```python
from build123d import *

# Parameters (mm, degrees)
SKETCH_1_W                = 35
SKETCH_1_H                = 10
EXTRUDE_1_DEPTH           = 30
SKETCH_2_R                = 1.65
CUT_EXTRUDE_1_DEPTH       = 47.368092477
SKETCH_3_W                = 35
SKETCH_3_H                = 10
FILLET_1_R                = 5
SKETCH_6_W                = 70
SKETCH_6_H                = 60
EXTRUDE_2_DEPTH           = 10
CHAMFER_1_SIZE            = 10
CUT_EXTRUDE_3_DEPTH       = 15
SKETCH_8_R                = 15
CUT_EXTRUDE_4_DEPTH       = 15
SKETCH_10_R               = 2.1
CUT_EXTRUDE_6_DEPTH       = 156.505811286
SKETCH_11_R               = 4.5
CUT_EXTRUDE_7_DEPTH       = 156.505811286
CUT_EXTRUDE_12_DEPTH      = 25
CUT_EXTRUDE_10_DEPTH      = 156.505811286
CUT_EXTRUDE_10_DEPTH_BACK = 156.505811286
SKETCH_14_W               = 35
SKETCH_14_H               = 27.103629711
SKETCH_15_W               = 35
SKETCH_15_H               = 10
EXTRUDE_3_DEPTH           = 23
CUT_EXTRUDE_11_DEPTH      = 164.332579917
CUT_EXTRUDE_11_DEPTH_BACK = 164.332579917
SKETCH_16_R               = 1.65
FILLET_2_R                = 3
CUT_EXTRUDE_START         = -4
CUT_EXTRUDE_13_DEPTH      = 4
SKETCH_19_W               = 35
SKETCH_19_H               = 24
EXTRUDE_4_DEPTH           = 6
CUT_EXTRUDE_14_DEPTH      = 162.92960956
CUT_EXTRUDE_14_DEPTH_BACK = 162.92960956
SKETCH_20_R               = 1.65
CUT_EXTRUDE_15_DEPTH      = 1
SKETCH_22_R               = 1.65
CUT_EXTRUDE_16_DEPTH      = 162.378361072
CUT_EXTRUDE_17_DEPTH      = 162.378361072
CUT_EXTRUDE_17_DEPTH_BACK = 162.378361072
SKETCH_25_R               = 1.25
CUT_EXTRUDE_18_DEPTH      = 10


with BuildPart() as part:
    # 草图1 → 凸台-拉伸1 (new body)
    with BuildSketch(Plane.XY):
        Rectangle(SKETCH_1_W, SKETCH_1_H)
    extrude(amount=EXTRUDE_1_DEPTH)

    # 草图2 → 切除-拉伸1 (cut, through all)
    with BuildSketch(Plane(origin=(17.5, 0, 0), x_dir=(0, 0, -1), z_dir=(1, 0, 0))):
        with Locations((-26, 0)):
            Circle(SKETCH_2_R)
        with Locations((-4, 0)):
            Circle(SKETCH_2_R)
    extrude(amount=-CUT_EXTRUDE_1_DEPTH, mode=Mode.SUBTRACT)

    # 扫描3: sweep along a path in 草图4
    with BuildLine(Plane(origin=(0, 0, 0), x_dir=(0, 0, -1), z_dir=(1, 0, 0))) as sweep_3_path:
        Line((-30, 0), (-31.113248654, 0))
        ThreePointArc((-31.113248654, 0), (-33.613248654, 0.669872981), (-35.443375673, 2.5))
        Line((-35.443375673, 2.5), (-99, 112.583302492))
    # 草图3 → 扫描3 (sweep)
    with BuildSketch(Plane.XY.offset(30)):
        Rectangle(SKETCH_3_W, SKETCH_3_H)
    sweep(path=sweep_3_path.line)

    # 圆角1
    fillet_1_edges = [part.edges().sort_by_distance(p)[0] for p in [
        (0, 5, 31.113248654),
    ]]
    fillet(fillet_1_edges, radius=FILLET_1_R)

    # 草图6 → 凸台-拉伸2 (add)
    with BuildSketch(Plane(origin=(0, -12.222431864, 21.169872981), x_dir=(-1, 0, 0), z_dir=(0, 0.4999999999999983, -0.8660254037844396))):
        with Locations((0, 117)):
            Rectangle(SKETCH_6_W, SKETCH_6_H)
    extrude(amount=-EXTRUDE_2_DEPTH)

    # 倒角1
    chamfer_1_edges = [part.edges().sort_by_distance(p)[0] for p in [
        (17.5, 60.621778265, 69),
        (-17.5, 60.621778265, 69),
    ]]
    chamfer(chamfer_1_edges, length=CHAMFER_1_SIZE)

    # 草图7 → 切除-拉伸3 (cut)
    with BuildSketch(Plane(origin=(0, -12.222431864, 21.169872981), x_dir=(-1, 0, 0), z_dir=(0, 0.4999999999999983, -0.8660254037844396))):
        with BuildLine():
            Line((-35, 147), (-35, 112))
            ThreePointArc((-35, 112), (-24.748737372, 136.748737311), (-8.6e-08, 147))
            Line((-8.6e-08, 147), (-35, 147))
        make_face()
        with BuildLine():
            ThreePointArc((-8.6e-08, 147), (24.748737311, 136.748737372), (35, 112))
            Line((35, 112), (35, 147))
            Line((35, 147), (-8.6e-08, 147))
        make_face()
    extrude(amount=-CUT_EXTRUDE_3_DEPTH, mode=Mode.SUBTRACT)

    # 草图8 → 切除-拉伸4 (cut)
    with BuildSketch(Plane(origin=(0, -12.222431864, 21.169872981), x_dir=(-1, 0, 0), z_dir=(0, 0.4999999999999983, -0.8660254037844396))):
        with Locations(Location((0, 112, 0), (0, 0, 90))):
            Circle(SKETCH_8_R)
    extrude(amount=-CUT_EXTRUDE_4_DEPTH, mode=Mode.SUBTRACT)

    # 草图10 → 切除-拉伸6 (cut, through all)
    with BuildSketch(Plane(origin=(0, -12.222431864, 21.169872981), x_dir=(-1, 0, 0), z_dir=(0, 0.4999999999999983, -0.8660254037844396))):
        with Locations(Location((0, 141, 0), (0, 0, 90))):
            Circle(SKETCH_10_R)
        with Locations(Location((-25.11473671, 97.5, 0), (0, 0, 90))):
            Circle(SKETCH_10_R)
        with Locations(Location((25.11473671, 97.5, 0), (0, 0, 90))):
            Circle(SKETCH_10_R)
    extrude(amount=-CUT_EXTRUDE_6_DEPTH, mode=Mode.SUBTRACT)

    # 草图11 → 切除-拉伸7 (cut, through all)
    with BuildSketch(Plane(origin=(0, -12.222431864, 21.169872981), x_dir=(-1, 0, 0), z_dir=(0, 0.4999999999999983, -0.8660254037844396))):
        with Locations((-16.670989023, 102.375)):
            Circle(SKETCH_11_R)
        with Locations((16.670989023, 102.375)):
            Circle(SKETCH_11_R)
    extrude(amount=-CUT_EXTRUDE_7_DEPTH, mode=Mode.SUBTRACT)

    # 草图12 → 切除-拉伸12 (cut)
    with BuildSketch(Plane(origin=(0, -12.222431864, 21.169872981), x_dir=(-1, 0, 0), z_dir=(0, 0.4999999999999983, -0.8660254037844396))):
        with BuildLine():
            Line((-20.682503653, 104.414056246), (-13.371715434, 118.796854152))
            ThreePointArc((-13.371715434, 118.796854152), (-12.990381057, 119.5), (-12.572106078, 120.181818182))
            Line((-12.572106078, 120.181818182), (-3.771631823, 133.704545455))
            ThreePointArc((-3.771631823, 133.704545455), (0, 135.75), (3.771631823, 133.704545455))
            Line((3.771631823, 133.704545455), (12.572106078, 120.181818182))
            ThreePointArc((12.572106078, 120.181818182), (12.990381057, 119.5), (13.371715434, 118.796854152))
            Line((13.371715434, 118.796854152), (20.682503653, 104.414056246))
            ThreePointArc((20.682503653, 104.414056246), (20.56810334, 100.125), (16.91087183, 97.8813983))
            Line((16.91087183, 97.8813983), (0.799609356, 97.021327666))
            ThreePointArc((0.799609356, 97.021327666), (0, 97), (-0.799609356, 97.021327666))
            Line((-0.799609356, 97.021327666), (-16.91087183, 97.8813983))
            ThreePointArc((-16.91087183, 97.8813983), (-20.56810334, 100.125), (-20.682503653, 104.414056246))
        make_face()
    extrude(amount=-CUT_EXTRUDE_12_DEPTH, mode=Mode.SUBTRACT)

    # 草图14 → 切除-拉伸10 (cut, two sides: drawn at the far end of the back side and taken through both)
    with BuildSketch(Plane(origin=(0, -12.222431864, 21.169872981), x_dir=(-1, 0, 0), z_dir=(0, 0.4999999999999983, -0.8660254037844396)).offset(-CUT_EXTRUDE_10_DEPTH_BACK)):
        with Locations((0, 9.221687837)):
            Rectangle(SKETCH_14_W, SKETCH_14_H)
    extrude(amount=CUT_EXTRUDE_10_DEPTH + CUT_EXTRUDE_10_DEPTH_BACK, mode=Mode.SUBTRACT)

    # 草图15 → 凸台-拉伸3 (add)
    with BuildSketch(Plane(origin=(0, 19.722431864, 11.386751346), x_dir=(1, 0, 0), z_dir=(0, -0.8660254037844397, -0.4999999999999984))):
        with Locations((0, 29.444863729)):
            Rectangle(SKETCH_15_W, SKETCH_15_H)
    extrude(amount=EXTRUDE_3_DEPTH)

    # 草图16 → 切除-拉伸11 (cut, two sides: drawn at the far end of the back side and taken through both)
    with BuildSketch(Plane(origin=(17.5, 0, 0), x_dir=(0, 0, -1), z_dir=(1, 0, 0)).offset(-CUT_EXTRUDE_11_DEPTH_BACK)):
        with Locations((-29.386751346, -7.990381057)):
            Circle(SKETCH_16_R)
        with Locations((-34.386751346, 0.669872981)):
            Circle(SKETCH_16_R)
    extrude(amount=CUT_EXTRUDE_11_DEPTH + CUT_EXTRUDE_11_DEPTH_BACK, mode=Mode.SUBTRACT)

    # 圆角2
    fillet_2_edges = [part.edges().sort_by_distance(p)[0] for p in [
        (-35, 60.621778265, 69),
        (35, 60.621778265, 69),
        (-17.5, 51.961524227, 64),
        (-27.5, 60.621778265, 69),
        (27.5, 60.621778265, 69),
        (17.5, 51.961524227, 64),
    ]]
    fillet(fillet_2_edges, radius=FILLET_2_R)

    # 草图18 → 切除-拉伸13 (cut)
    with BuildSketch(Plane(origin=(0, -12.222431864, 21.169872981), x_dir=(-1, 0, 0), z_dir=(0, 0.4999999999999983, -0.8660254037844396)).offset(CUT_EXTRUDE_START)):
        with BuildLine():
            Line((-17.5, 75.757359313), (17.5, 75.757359313))
            ThreePointArc((17.5, 75.757359313), (17.728361402, 76.90540961), (18.378679656, 77.878679656))
            Line((18.378679656, 77.878679656), (26.621320344, 86.121320344))
            ThreePointArc((26.621320344, 86.121320344), (27.59459039, 86.771638598), (28.742640687, 87))
            Line((28.742640687, 87), (32, 87))
            ThreePointArc((32, 87), (34.121320344, 87.878679656), (35, 90))
            Line((35, 90), (35, 112))
            ThreePointArc((35, 112), (0, 147), (-35, 112))
            Line((-35, 112), (-35, 90))
            ThreePointArc((-35, 90), (-34.121320344, 87.878679656), (-32, 87))
            Line((-32, 87), (-28.742640687, 87))
            ThreePointArc((-28.742640687, 87), (-27.59459039, 86.771638598), (-26.621320344, 86.121320344))
            Line((-26.621320344, 86.121320344), (-18.378679656, 77.878679656))
            ThreePointArc((-18.378679656, 77.878679656), (-17.728361402, 76.90540961), (-17.5, 75.757359313))
        make_face()
    extrude(amount=CUT_EXTRUDE_13_DEPTH, mode=Mode.SUBTRACT)

    # 草图19 → 凸台-拉伸4 (add)
    with BuildSketch(Plane(origin=(0, -12.222431864, 21.169872981), x_dir=(-1, 0, 0), z_dir=(0, 0.4999999999999983, -0.8660254037844396))):
        with Locations((0, 11.773502692)):
            Rectangle(SKETCH_19_W, SKETCH_19_H)
    extrude(amount=EXTRUDE_4_DEPTH)

    # 草图20 → 切除-拉伸14 (cut, two sides: drawn at the far end of the back side and taken through both)
    with BuildSketch(Plane.ZY.offset(17.5).offset(-CUT_EXTRUDE_14_DEPTH_BACK)):
        with Locations(Location((29.386751346, -7.990381057, 0), (0, 0, 180))):
            Circle(SKETCH_20_R)
        with Locations(Location((34.386751346, 0.669872981, 0), (0, 0, 180))):
            Circle(SKETCH_20_R)
        with Locations((22.458548116, -3.990381057)):
            Circle(SKETCH_20_R)
        with Locations((27.458548116, 4.669872981)):
            Circle(SKETCH_20_R)
    extrude(amount=CUT_EXTRUDE_14_DEPTH + CUT_EXTRUDE_14_DEPTH_BACK, mode=Mode.SUBTRACT)

    # 草图21 → 切除-拉伸15 (cut)
    with BuildSketch(Plane(origin=(0, -17.222431864, 29.830127019), x_dir=(1, 0, 0), z_dir=(0, -0.4999999999999983, 0.8660254037844396))):
        with BuildLine():
            Line((-35, 112), (-35, 90))
            ThreePointArc((-35, 90), (-34.121320344, 87.878679656), (-32, 87))
            Line((-32, 87), (-28.742640687, 87))
            ThreePointArc((-28.742640687, 87), (-27.59459039, 86.771638598), (-26.621320344, 86.121320344))
            Line((-26.621320344, 86.121320344), (-18.378679656, 77.878679656))
            ThreePointArc((-18.378679656, 77.878679656), (-17.728361402, 76.90540961), (-17.5, 75.757359313))
            Line((-17.5, 75.757359313), (-17.5, -0.226497308))
            Line((-17.5, -0.226497308), (17.5, -0.226497308))
            Line((17.5, -0.226497308), (17.5, 75.757359313))
            ThreePointArc((17.5, 75.757359313), (17.728361402, 76.90540961), (18.378679656, 77.878679656))
            Line((18.378679656, 77.878679656), (26.621320344, 86.121320344))
            ThreePointArc((26.621320344, 86.121320344), (27.59459039, 86.771638598), (28.742640687, 87))
            Line((28.742640687, 87), (32, 87))
            ThreePointArc((32, 87), (34.121320344, 87.878679656), (35, 90))
            Line((35, 90), (35, 112))
            ThreePointArc((35, 112), (0, 147), (-35, 112))
        make_face()
    extrude(amount=-CUT_EXTRUDE_15_DEPTH, mode=Mode.SUBTRACT)

    # 草图22 → 切除-拉伸16 (cut, through all)
    with BuildSketch(Plane.ZY.offset(17.5)):
        with Locations((49.386751346, 26.650635095)):
            Circle(SKETCH_22_R)
        with Locations((56.886751346, 39.641016151)):
            Circle(SKETCH_22_R)
        with Locations((41.886751346, 13.660254038)):
            Circle(SKETCH_22_R)
    extrude(amount=-CUT_EXTRUDE_16_DEPTH, mode=Mode.SUBTRACT)

    # 草图23 → 切除-拉伸17 (cut, two sides: drawn at the far end of the back side and taken through both)
    with BuildSketch(Plane(origin=(17.5, 0, 0), x_dir=(0, 0, -1), z_dir=(1, 0, 0)).offset(-CUT_EXTRUDE_17_DEPTH_BACK)):
        Polygon((-59.048552638, 53.385365824), (-21.056624327, -12.418584287), (-8.944037263, -5.425378885), align=None)
    extrude(amount=CUT_EXTRUDE_17_DEPTH + CUT_EXTRUDE_17_DEPTH_BACK, mode=Mode.SUBTRACT)

    # 草图25 → 切除-拉伸18 (cut)
    with BuildSketch(Plane(origin=(0, -12.222431864, 21.169872981), x_dir=(-1, 0, 0), z_dir=(0, 0.4999999999999981, -0.8660254037844397))):
        with Locations(Location((-9, 58.973502692, 0), (0, 0, 90))):
            Circle(SKETCH_25_R)
        with Locations(Location((9, 58.973502692, 0), (0, 0, 90))):
            Circle(SKETCH_25_R)
        with Locations(Location((-9, 13.773502692, 0), (0, 0, 90))):
            Circle(SKETCH_25_R)
        with Locations(Location((9, 13.773502692, 0), (0, 0, 90))):
            Circle(SKETCH_25_R)
    extrude(amount=-CUT_EXTRUDE_18_DEPTH, mode=Mode.SUBTRACT)


solid = part.part
```
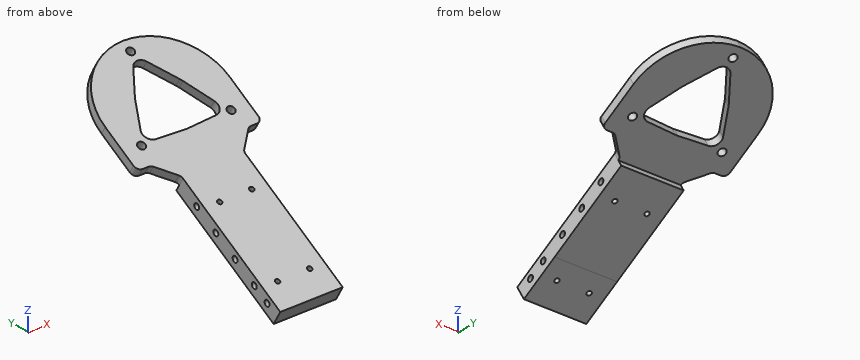
Here's how the part is built. I have some questions about the finished solid (model axes, mm). Round coordinates to 2 decimals unless told otherwise and drop trailing zeros. Write each loop counter-clockwise with the first axis right and the second up, starting at its lowest first coordinate (ties: lowest second). Pieces come first, ordered by that corner, then holes. Notation, with made-up numbers: M 85,-17 L 111,-17 A8 cw 111,-4 Z; hole C 83.5,4 d1. An arc over 180 degrees is marked long. Answer as CSV lines item,"result". Start each with the question number.
1. Suppose I cut it at A-A on z = 26. Write out the boundary of the cut face in (x, y).
2. I'm going to push flat-ended pins straight in: pin 1 Ø5.5 at (y, z) = (26.65, 49.39) entering from +X; pin 2 Ø5.5 at (y, z) = (0.67, 34.39) entering from -X; pin 3 Ø8 at (x, y) = (2.5, 19.5) entering from -Z. Where does each tip first touch, or does it pass through?
3. Suppose I cut it at B-B on y = 31.5. Write out the boundary of the cut face in (x, z), then the cut area to 3 significant figures.
4. I need wall thicknesses on probe 1 along Z at (x, y) = (-4, 0.5); probe 2 along Y at (x, z) = (13.5, 33.5); probe 3 along Z at (x, y) = (-15.5, 51.5). Which ranges of each line are inside material? Lowest first, please.
Check result:
1,outline,"M -17.5,-15.27 L 17.5,-15.27 L 17.5,-3.86 L -17.5,-3.86 Z"
2,pin 1,"stops at x = 17.5"
2,pin 2,"stops at x = -17.5"
2,pin 3,"stops at z = 37.18"
3,outline,"M -17.5,46.41 L 17.5,46.41 L 17.5,56.81 L -17.5,56.81 Z"
3,area,"364 mm2"
4,probe 1,"z = 28.52 to 32.75, 36.03 to 38.91"
4,probe 2,"y = -8.87 to -0.72, 2.06 to 9.13"
4,probe 3,"z = 57.96 to 62.31, 62.58 to 68.35"
